from build123d import *

# Parameters (mm, degrees)
SKETCH1_R                                           = 50
SKETCH1_R_2                                         = 20.25
BOSS_EXTRUDE1_DEPTH                                 = 6
CBORE_FOR_M3_HEX_SOCKET_HEAD_CAP_SCREW2_D           = 3.4
CBORE_FOR_M3_HEX_SOCKET_HEAD_CAP_SCREW2_CBORE_D     = 6.5
CBORE_FOR_M3_HEX_SOCKET_HEAD_CAP_SCREW2_CBORE_DEPTH = 3.4
BOSS_EXTRUDE2_START                                 = -6
BOSS_EXTRUDE2_DEPTH                                 = 6
BOSS_EXTRUDE3_START                                 = -6
BOSS_EXTRUDE3_DEPTH                                 = 6
CBORE_FOR_M3_HEX_SOCKET_HEAD_CAP_SCREW1_D           = 3.4
CBORE_FOR_M3_HEX_SOCKET_HEAD_CAP_SCREW1_CBORE_D     = 6.5
CBORE_FOR_M3_HEX_SOCKET_HEAD_CAP_SCREW1_CBORE_DEPTH = 3.4
CUT_EXTRUDE1_DEPTH                                  = 3.4
FILLET1_R                                           = 1
TAP_DRILL_FOR_M6_HELICOIL1_D                        = 6.25


with BuildPart() as part:
    # Sketch1 → Boss-Extrude1 (new body)
    with BuildSketch(Plane(origin=(0, 0, 0), x_dir=(1, 0, 0), z_dir=(0, 1, 0))):
        with Locations(Location((0, 0, 0), (0, 0, 270))):
            Circle(SKETCH1_R)
        with Locations(Location((0, 0, 0), (0, 0, 270))):
            Circle(SKETCH1_R_2, mode=Mode.SUBTRACT)
    extrude(amount=BOSS_EXTRUDE1_DEPTH)

    # CBORE for M3 Hex Socket Head Cap Screw2 (through all)
    with Locations(Plane(origin=(0, 6, 0), x_dir=(1, 0, 0), z_dir=(0, 1, 0))):
        with Locations((-40.696782834, 12.248341396), (-20.116085855, 37.437856374), (12.248341396, 40.696782834), (37.437856374, 20.116085855), (40.696782834, -12.248341396), (20.116085855, -37.437856374), (-12.248341396, -40.696782834), (-37.437856374, -20.116085855)):
            CounterBoreHole(CBORE_FOR_M3_HEX_SOCKET_HEAD_CAP_SCREW2_D / 2, CBORE_FOR_M3_HEX_SOCKET_HEAD_CAP_SCREW2_CBORE_D / 2, CBORE_FOR_M3_HEX_SOCKET_HEAD_CAP_SCREW2_CBORE_DEPTH)

    # Sketch6 → Boss-Extrude2 (add)
    with BuildSketch(Plane(origin=(0, 6, 0), x_dir=(1, 0, 0), z_dir=(0, 1, 0)).offset(BOSS_EXTRUDE2_START)):
        with BuildLine():
            Line((-50, 0), (-50, -60))
            Line((-50, -60), (50, -60))
            Line((50, -60), (50, 0))
            ThreePointArc((50, 0), (0, -50), (-50, 0))
        make_face()
    extrude(amount=BOSS_EXTRUDE2_DEPTH)

    # Sketch10 → Boss-Extrude3 (add)
    with BuildSketch(Plane(origin=(0, 6, 0), x_dir=(1, 0, 0), z_dir=(0, 1, 0)).offset(BOSS_EXTRUDE3_START)):
        with BuildLine():
            Line((-50, 0), (-50, 60))
            Line((-50, 60), (50, 60))
            Line((50, 60), (50, 0))
            ThreePointArc((50, 0), (0, 50), (-50, 0))
        make_face()
    extrude(amount=BOSS_EXTRUDE3_DEPTH)

    # CBORE for M3 Hex Socket Head Cap Screw1 (through all)
    with Locations(Plane(origin=(0, 6, 0), x_dir=(1, 0, 0), z_dir=(0, 1, 0))):
        with Locations((-40, 57), (-20, 57), (0, 57), (20, 57), (40, 57), (40, -57), (20, -57), (0, -57), (-20, -57), (-40, -57)):
            CounterBoreHole(CBORE_FOR_M3_HEX_SOCKET_HEAD_CAP_SCREW1_D / 2, CBORE_FOR_M3_HEX_SOCKET_HEAD_CAP_SCREW1_CBORE_D / 2, CBORE_FOR_M3_HEX_SOCKET_HEAD_CAP_SCREW1_CBORE_DEPTH)

    # Sketch13 → Cut-Extrude1 (cut)
    with BuildSketch(Plane(origin=(0, 6, 0), x_dir=(1, 0, 0), z_dir=(0, 1, 0))):
        with BuildLine():
            Line((-43.25, 57), (-43.25, 60))
            Line((-43.25, 60), (-36.75, 60))
            Line((-36.75, 60), (-36.75, 57))
            ThreePointArc((-36.75, 57), (-40, 53.75), (-43.25, 57))
        make_face()
        with BuildLine():
            Line((-23.25, 57), (-23.25, 60))
            Line((-23.25, 60), (-16.75, 60))
            Line((-16.75, 60), (-16.75, 57))
            ThreePointArc((-16.75, 57), (-20, 53.75), (-23.25, 57))
        make_face()
        with BuildLine():
            Line((-3.25, 57), (-3.25, 60))
            Line((-3.25, 60), (3.25, 60))
            Line((3.25, 60), (3.25, 57))
            ThreePointArc((3.25, 57), (0, 53.75), (-3.25, 57))
        make_face()
        with BuildLine():
            Line((16.75, 57), (16.75, 60))
            Line((16.75, 60), (23.25, 60))
            Line((23.25, 60), (23.25, 57))
            ThreePointArc((23.25, 57), (20, 53.75), (16.75, 57))
        make_face()
        with BuildLine():
            Line((36.75, 57), (36.75, 60))
            Line((36.75, 60), (43.25, 60))
            Line((43.25, 60), (43.25, 57))
            ThreePointArc((43.25, 57), (40, 53.75), (36.75, 57))
        make_face()
        with BuildLine():
            Line((43.25, -60), (43.25, -57))
            ThreePointArc((43.25, -57), (40, -53.75), (36.75, -57))
            Line((36.75, -57), (36.75, -60))
            Line((36.75, -60), (43.25, -60))
        make_face()
        with BuildLine():
            Line((23.25, -60), (23.25, -57))
            ThreePointArc((23.25, -57), (20, -53.75), (16.75, -57))
            Line((16.75, -57), (16.75, -60))
            Line((16.75, -60), (23.25, -60))
        make_face()
        with BuildLine():
            Line((3.25, -60), (3.25, -57))
            ThreePointArc((3.25, -57), (0, -53.75), (-3.25, -57))
            Line((-3.25, -57), (-3.25, -60))
            Line((-3.25, -60), (3.25, -60))
        make_face()
        with BuildLine():
            Line((-16.75, -60), (-16.75, -57))
            ThreePointArc((-16.75, -57), (-20, -53.75), (-23.25, -57))
            Line((-23.25, -57), (-23.25, -60))
            Line((-23.25, -60), (-16.75, -60))
        make_face()
        with BuildLine():
            Line((-36.75, -60), (-36.75, -57))
            ThreePointArc((-36.75, -57), (-40, -53.75), (-43.25, -57))
            Line((-43.25, -57), (-43.25, -60))
            Line((-43.25, -60), (-36.75, -60))
        make_face()
    extrude(amount=-CUT_EXTRUDE1_DEPTH, mode=Mode.SUBTRACT)

    # Fillet1
    fillet1_edges = [part.edges().sort_by_distance(p)[0] for p in [
        (-36.75, 4.3, 60),
        (-43.25, 4.3, 60),
        (-16.75, 4.3, 60),
        (-23.25, 4.3, 60),
        (3.25, 4.3, 60),
        (-3.25, 4.3, 60),
        (23.25, 4.3, 60),
        (16.75, 4.3, 60),
        (43.25, 4.3, 60),
        (36.75, 4.3, 60),
        (36.75, 4.3, -60),
        (43.25, 4.3, -60),
        (16.75, 4.3, -60),
        (23.25, 4.3, -60),
        (-3.25, 4.3, -60),
        (3.25, 4.3, -60),
        (-23.25, 4.3, -60),
        (-16.75, 4.3, -60),
        (-43.25, 4.3, -60),
        (-36.75, 4.3, -60),
        (50, 3, 60),
        (-50, 3, 60),
        (-50, 3, -60),
        (50, 3, -60),
    ]]
    fillet(fillet1_edges, radius=FILLET1_R)

    # Tap Drill for M6 Helicoil1 (through all)
    with Locations(Plane(origin=(0, 6, 0), x_dir=(1, 0, 0), z_dir=(0, 1, 0))):
        with Locations((31.819805153, -31.819805153), (31.819805153, 31.819805153), (-31.819805153, -31.819805153), (-31.819805153, 31.819805153), (0, 0)):
            Hole(TAP_DRILL_FOR_M6_HELICOIL1_D / 2)


solid = part.part
CAD build for the part. Positions are in the model's coordinates, mm. A direction names the side the tool comes from. Round coordinates to 2 decimals unless told otherwise and drop trailing zeros. Order: outer loops, then holes, each group sorted by start corner. A loop starts at its lowest first (then second) coordinate and runs counter-clockwise, first axis right, second up. Notation, with made-up numbers: (-28, 80) - (3, 80) arc R25 cw to (3, 93) - close; hole circle Ø10 at (15.25, 89). An arc over 180 degrees is marked (long way). Return JSON: item names as keys, results as strings.
(1) Cut at C-C (y = 3.85). State how many separate pieces and enclosed holes the cut face has, then the cut area to 3 significant figures.
Answer key:
{"separate pieces": "1", "enclosed holes": "13", "area": "9,960 mm^2"}
(2) Cut at B-B (x = -6.5). Give the cut face in (y, z), then the cut area to 3 significant figures.
Answer key:
{"outline": "(0, -60) - (6, -60) - (6, -19.18) - (0, -19.18) - close; (0, 19.18) - (6, 19.18) - (6, 60) - (0, 60) - close", "area": "490 mm^2"}
(3) Pull direction Z, two halves, no side cores. Call faces 6 (the face through (-10.501, 4.324, 37.956)), 7 (the face through (0, 2.6, 59)), 8 (the face through (-19.93, 4.32, 53.75)): +Z half, -Z half, draft (parallel to the pull), parting line (faces both ways), or undercut.
Answer key:
{"face 6": "undercut", "face 7": "draft", "face 8": "+Z half"}
(4) Pin check, flat tip, straight feed: pin 1 Ø5.5 at (x, z) = (40, 57) entering from +Y. Stop position of the tip, or through.
Answer key:
{"pin 1": "stops at y = 2.6"}
(5) Wall check: probe 1 along Z at (x, y) = (21, 0.85); probe 2 along X at (y, z) = (2.85, -34.5); probe 3 along X at (y, z) = (1.35, 0). Give the ranges that are in metal, low to high. Write a range as from..to.
Answer key:
{"probe 1": "z = -60..-58.37, -55.63..35.99, 38.89..55.63, 58.37..60", "probe 2": "x = -50..-33.43, -30.21..-21.51, -18.73..30.21, 33.43..50", "probe 3": "x = -50..-20.25, 20.25..50"}
(6) Cut at A-A (z = 0). Give the cut face in (x, y), then the cut area to 3 significant figures.
Answer key:
{"outline": "(-50, 0) - (-20.25, 0) - (-20.25, 6) - (-50, 6) - close; (20.25, 0) - (50, 0) - (50, 6) - (20.25, 6) - close", "area": "357 mm^2"}
(7) Tool access for faces 1 (the face through (-20, 2.6, 59)), 2 (the face through (-40, 2.6, -59)), 3 (the face through (-22, 0, -1)), 4 (the face through (21.863, 4.324, 34.697)), 5 (the face through (-20.914, 1.282, -58.433)): list every direction of +Z, -Z, +X, -X, +Y, -Y with a clear straight run to the whole face (end or side of a thin tool).
Answer key:
{"face 1": "+Z, +Y", "face 2": "-Z, +Y", "face 3": "+Z, -Z, +X, -X, -Y", "face 4": "+Y", "face 5": "+Y, -Y"}
